```python
from build123d import *

# Parameters (mm, degrees)
SKETCH_1_R      = 1.5
SKETCH_1_W      = 2.85
SKETCH_1_H      = 5
EXTRUDE_1_DEPTH = 1.4


with BuildPart() as part:
    # Эскиз1 → Бобышка-Вытянуть1 (new, symmetric)
    with BuildSketch(Plane.XY):
        with BuildLine():
            ThreePointArc((175.091334091, 16.644787515), (168.620686799, 13.96455765), (165.940456932, 7.493910359))
            ThreePointArc((165.940456932, 7.493910359), (168.620686797, 1.023263065), (175.091334091, -1.656966802))
            add(Edge.make_bspline(
                [(175.091334091, -1.656966802), (177.330680613, -1.588466601), (181.854695323, -1.455127256), (188.663234462, -1.270383377), (195.516645168, -1.101112884), (202.369532894, -0.948617189), (211.49919029, -0.767742353), (220.603098666, -0.619939742), (229.617630172, -0.50292618), (236.087353854, -0.431514192), (241.980776913, -0.376520461), (246.558970011, -0.339535886), (249.120490965, -0.321271242), (250, -0.315)],
                knots=[0.704401069, 0.704401069, 0.704401069, 0.704401069, 0.730918775, 0.757971338, 0.785017763, 0.812061651, 0.839103366, 0.893099152, 0.919831065, 0.945809917, 0.969680601, 0.989589706, 1, 1, 1, 1], degree=3))
            ThreePointArc((250, -0.315), (250.130477272, 0), (250, 0.315))
            add(Edge.make_bspline(
                [(250, 0.315), (249.15566774, 0.545019818), (246.720175698, 1.208516243), (242.391332083, 2.358339053), (236.849761204, 3.787625364), (230.779918279, 5.298008837), (224.455917947, 6.812866028), (218.030543496, 8.291610632), (211.562405045, 9.719735057), (205.072411509, 11.092374932), (198.567970913, 12.407850726), (192.052369914, 13.665297924), (185.527619973, 14.864093303), (179.872800983, 15.850364437), (176.392239334, 16.431323122), (175.091334091, 16.644787515)],
                knots=[0, 0, 0, 0, 0.0101622, 0.029313053, 0.052011605, 0.076619468, 0.101948061, 0.127526132, 0.153184131, 0.178867888, 0.204557903, 0.230245712, 0.255925967, 0.281594302, 0.296903142, 0.296903142, 0.296903142, 0.296903142], degree=3))
        make_face()
        with Locations((175.091334091, 7.493910357)):
            Circle(SKETCH_1_R, mode=Mode.SUBTRACT)
        with Locations((205.091334091, 4.493910357)):
            Rectangle(SKETCH_1_W, SKETCH_1_H, mode=Mode.SUBTRACT)
    extrude(amount=EXTRUDE_1_DEPTH, both=True)


solid = part.part
```
Verification items for the finished model (mm, model axes). A direction names the side the tool comes from. Round coordinates to 2 decimals unless told otherwise and drop trailing zeros. Order: outer loops, then holes, each group sorted by start corner. A loop starts at its lowest first (then second) coordinate and runs counter-clockwise, first axis right, second up.
1) Depth check by flat-ended pin: pin 1 (1.4 mm diameter, centred on y = 5, z = -0.5, fed in from -X). Enter the tip coordinate at first touch or a pass-through.
Geometry says:
pin 1: stops at x = 166.12
2) Cross-section at B-B, the plane z = -0.55. Give the number of separate pieces and of enclosed holes in the cut face, plus the area to 3 significant figures.
Geometry says:
separate pieces: 1
enclosed holes: 2
area: 859 mm2
3) Draft check along Y on faces 1 (the flat face through (203.666, 4, 0)), 2 (the cylindrical face through (165.943, 7.695, 0.02)), 3 (the flat face through (198, 6, 1.4)). Enter one of: +Y half, -Y half, draft (parallel to the pull), parting line (faces both ways), or undercut.
Geometry says:
face 1: undercut
face 2: parting line
face 3: draft
4) Tool access check on faces 4 (the flat face through (205, 6.994, 0)), 5 (the flat face through (198, 6, -1.4)). Record the directions out of +Z, -Z, +X, -X, +Y, -Y that give a thin tool (end or side, any length) a straight path to the whole face; none if there is none.
Geometry says:
face 4: +Z, -Z
face 5: -Z, +X, -X, +Y, -Y
5) Material ranges on line 1 (Y direction, x = 183, z = -0.45); line 2 (Y direction, x = 187.5, z = -0.25), recorded low to high.
Geometry says:
line 1: y = -1.43 to 15.3
line 2: y = -1.3 to 14.5
6) Cross-section at A-A, the plane x = 172. Record the cut outline in (y, z).
Geometry says:
outline: (-1.12, -1.4) - (16.11, -1.4) - (16.11, 1.4) - (-1.12, 1.4) - close
